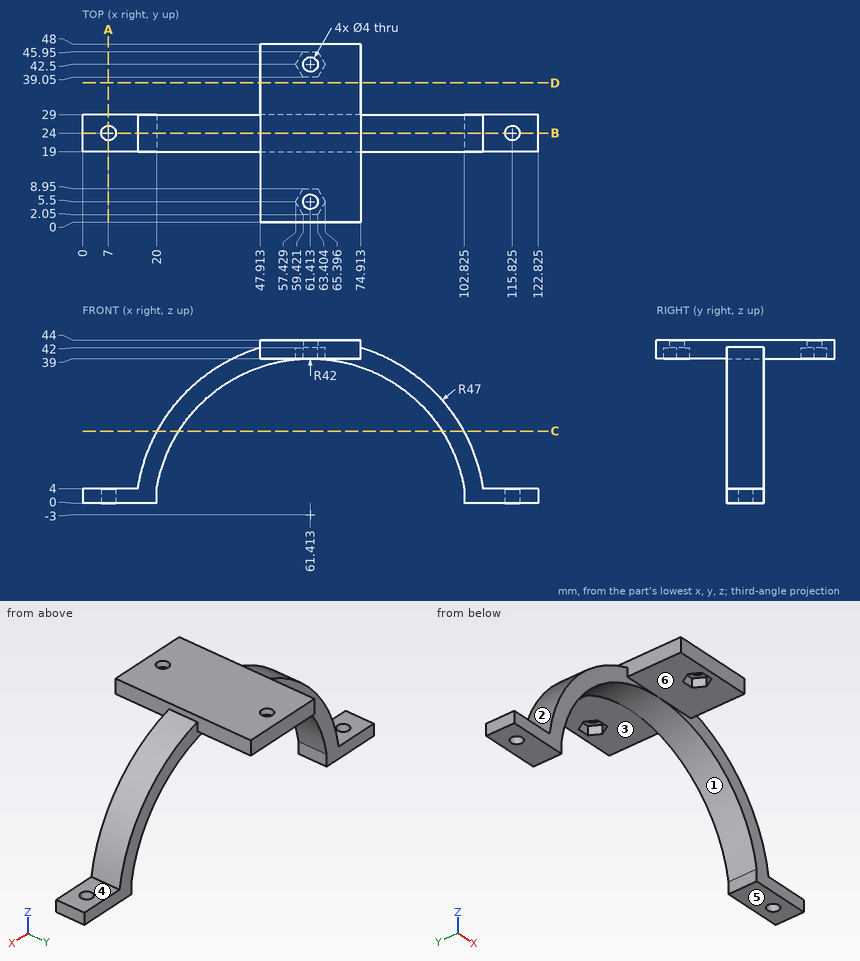
Study the drawing (mm; zero at the part's minimum x, y, z) and answer. A direction names the side the tool comes from. Give positions to 0.01 mm unless a question says otherwise; leave off trailing zeros. Write each loop counter-clockwise with the first axis right and the second up, starting at its lowest first coordinate (ties: lowest second). Pieces come first, ordered by that corner, then holes. Notation, with made-up numbers: (5.5, 29.5) - (9.5, 29.5) arc R14 ccw to (9.5, 54.5) - close; hole circle Ø9 at (-27.75, -38). An arc over 180 degrees is marked (long way). Write item = value, one per line. Start each with the question number.
Item 1: A tool of negligible diameter and unlimited length cuts with its end or side. For the marked faces 4, 5 and 6, from which of +Z, -Z, +X, -X, +Y, -Y can it reach the whole face along a straight path? Write none if from no direction.
Item 2: The mould has two halves that part along X. Classify the marked faces 1, 2 and 3: +X half, -X half, draft (parallel to the pull), parting line (faces both ways), or undercut.
Item 3: Each of these flat-tipped pins is pushed along its axis until it touches: P1, Ø21, axis at x = 64, y = 38, coming from the -Z side; P2, Ø15, axis at x = 67.5, y = 9, coming from the -Z side; P3, Ø11, axis at x = 4, y = 21.5, coming from the +Z side; P4, Ø3.5, axis at x = 60.5, z = 41, coming from the -Y side. Where does it stop, or does it pass through?
Item 4: Find section A-A (x = 7). Give the vertices of the cut face in (y, z).
Item 5: Find section B-B (y = 24). Give the vertices of the cut face in (x, z) (1 decimal).
Item 6: Find section C-C (z = 19.5). Give the vertices of the cut face in (x, y), then the cut area to 3 significant figures.
Item 7: Find section D-D (y = 37.5). Give the vertices of the cut face in (x, z), then the cut area to 3 significant figures.
Item 8: Find the intervals of material crossed by probe 1 along Y at (x, z) = (7, 1.7); probe 2 along Z at (x, y) = (64.5, 11); probe 3 along Y at (x, z) = (83.5, 38), in increasing order. Write a range as [from, to].
Response:
q1.face_4 = +Z, +X, +Y, -Y
q1.face_5 = -Z, +X, -X, +Y, -Y
q1.face_6 = -Z, +X, -X, -Y
q2.face_1 = undercut
q2.face_2 = -X half
q2.face_3 = draft
q3.P1 = 38.23
q3.P2 = 39
q3.P3 = 4
q3.P4 = 0
q4.outline = (19, 0) - (22, 0) - (22, 4) - (19, 4) - close; (26, 0) - (29, 0) - (29, 4) - (26, 4) - close
q5.outline = (0, 0) - (5, 0) - (5, 4) - (0, 4) - close; (9, 0) - (20, 0) - (20, 4) arc R42 cw to (102.8, 4) - (102.8, 0) - (113.8, 0) - (113.8, 4) - (107.9, 4) arc R47 ccw to (74.9, 42) - (74.9, 44) - (47.9, 44) - (47.9, 42) arc R47 ccw to (14.9, 4) - (9, 4) - close; (117.8, 0) - (122.8, 0) - (122.8, 4) - (117.8, 4) - close
q6.outline = (20.15, 19) - (25.95, 19) - (25.95, 29) - (20.15, 29) - close; (96.88, 19) - (102.68, 19) - (102.68, 29) - (96.88, 29) - close
q6.area = 116 mm²
q7.outline = (47.91, 39) - (74.91, 39) - (74.91, 44) - (47.91, 44) - close
q7.area = 135 mm²
q8.probe_1 = [19, 22], [26, 29]
q8.probe_2 = [39, 44]
q8.probe_3 = [19, 29]
